from build123d import *

# Parameters (mm, degrees)
SKETCH1_W           = 32.9
SKETCH1_H           = 22.4
BOSS_EXTRUDE1_DEPTH = 5
SKETCH2_R           = 1.2
SKETCH2_W           = 22.9
SKETCH2_H           = 12.4
CUT_EXTRUDE2_DEPTH  = 5
SKETCH3_W           = 22.996888994
SKETCH3_H           = 5
BOSS_EXTRUDE2_DEPTH = 12.3
SKETCH4_R           = 1.2
CUT_EXTRUDE3_DEPTH  = 5
SKETCH6_W           = 5
SKETCH6_H           = 5
SKETCH6_W_2         = 4.903111006
BOSS_EXTRUDE3_DEPTH = 12.3
SKETCH8_W           = 17.3
SKETCH8_H           = 4.998204887
BOSS_EXTRUDE4_DEPTH = 3.1
SKETCH9_W           = 17.3
SKETCH9_H           = 5
BOSS_EXTRUDE5_DEPTH = 3.1
SKETCH18_W          = 5
SKETCH18_H          = 12.4
BOSS_EXTRUDE7_DEPTH = 30
SKETCH19_R          = 4.5
CUT_EXTRUDE6_DEPTH  = 30
SKETCH20_R          = 4.5
CUT_EXTRUDE7_DEPTH  = 30
SKETCH10_W          = 5
SKETCH10_H          = 12.4
BOSS_EXTRUDE6_DEPTH = 30
SKETCH21_R          = 4.5
CUT_EXTRUDE8_DEPTH  = 10
SKETCH22_R          = 4.5
CUT_EXTRUDE9_DEPTH  = 10


with BuildPart() as part:
    # Sketch1 → Boss-Extrude1 (new body)
    with BuildSketch(Plane.XY):
        Rectangle(SKETCH1_W, SKETCH1_H)
    extrude(amount=BOSS_EXTRUDE1_DEPTH)

    # Sketch2 → Cut-Extrude2 (cut)
    with BuildSketch(Plane.XY.offset(5)):
        with Locations((13.8, 0)):
            Circle(SKETCH2_R)
        with Locations((-13.8, 0)):
            Circle(SKETCH2_R)
        Rectangle(SKETCH2_W, SKETCH2_H)
    extrude(amount=-CUT_EXTRUDE2_DEPTH, mode=Mode.SUBTRACT)

    # Sketch3 → Boss-Extrude2 (add)
    with BuildSketch(Plane.XY.offset(5)):
        with Locations((0.048444497, 8.7)):
            Rectangle(SKETCH3_W, SKETCH3_H)
        with Locations((0.048444497, -8.7)):
            Rectangle(SKETCH3_W, SKETCH3_H)
    extrude(amount=BOSS_EXTRUDE2_DEPTH)

    # Sketch4 → Cut-Extrude3 (cut)
    with BuildSketch(Plane.XY.offset(17.3)):
        with Locations((0.048444497, 8.7)):
            Circle(SKETCH4_R)
        with Locations((0.048444497, -8.7)):
            Circle(SKETCH4_R)
    extrude(amount=-CUT_EXTRUDE3_DEPTH, mode=Mode.SUBTRACT)

    # Sketch6 → Boss-Extrude3 (add)
    with BuildSketch(Plane.XY.offset(5)):
        with Locations((-13.95, -8.7)):
            Rectangle(SKETCH6_W, SKETCH6_H)
        with Locations((13.998444497, -8.7)):
            Rectangle(SKETCH6_W_2, SKETCH6_H)
    extrude(amount=BOSS_EXTRUDE3_DEPTH)

    # Sketch8 → Boss-Extrude4 (add)
    with BuildSketch(Plane(origin=(16.45, 0, 0), x_dir=(0, 0, -1), z_dir=(1, 0, 0))):
        with Locations((-8.65, -8.700897557)):
            Rectangle(SKETCH8_W, SKETCH8_H)
    extrude(amount=BOSS_EXTRUDE4_DEPTH)

    # Sketch9 → Boss-Extrude5 (add)
    with BuildSketch(Plane.ZY.offset(16.45)):
        with Locations((8.65, -8.7)):
            Rectangle(SKETCH9_W, SKETCH9_H)
    extrude(amount=BOSS_EXTRUDE5_DEPTH)

    # Sketch18 → Boss-Extrude7 (add)
    with BuildSketch(Plane.XZ.offset(11.2)):
        with Locations((-17.05, 8.65)):
            Rectangle(SKETCH18_W, SKETCH18_H)
        with Locations((17.05, 8.65)):
            Rectangle(SKETCH18_W, SKETCH18_H)
    extrude(amount=BOSS_EXTRUDE7_DEPTH)

    # Sketch19 → Cut-Extrude6 (cut)
    with BuildSketch(Plane.ZY.offset(19.55)):
        with Locations((8.65, -34.8)):
            Circle(SKETCH19_R)
    extrude(amount=-CUT_EXTRUDE6_DEPTH, mode=Mode.SUBTRACT)

    # Sketch20 → Cut-Extrude7 (cut)
    with BuildSketch(Plane(origin=(19.55, 0, 0), x_dir=(0, 0, -1), z_dir=(1, 0, 0))):
        with Locations((-8.65, -34.8)):
            Circle(SKETCH20_R)
    extrude(amount=-CUT_EXTRUDE7_DEPTH, mode=Mode.SUBTRACT)

    # Sketch10 → Boss-Extrude6 (add)
    with BuildSketch(Plane.XZ.offset(11.2)):
        with Locations((17.05, 8.65)):
            Rectangle(SKETCH10_W, SKETCH10_H)
        with Locations((-17.05, 8.65)):
            Rectangle(SKETCH10_W, SKETCH10_H)
    extrude(amount=BOSS_EXTRUDE6_DEPTH)

    # Sketch21 → Cut-Extrude8 (cut)
    with BuildSketch(Plane(origin=(19.55, 0, 0), x_dir=(0, 0, -1), z_dir=(1, 0, 0))):
        with Locations((-8.65, -34.8)):
            Circle(SKETCH21_R)
    extrude(amount=-CUT_EXTRUDE8_DEPTH, mode=Mode.SUBTRACT)

    # Sketch22 → Cut-Extrude9 (cut)
    with BuildSketch(Plane(origin=(-14.55, 0, 0), x_dir=(0, 0, -1), z_dir=(1, 0, 0))):
        with Locations((-8.65, -34.8)):
            Circle(SKETCH22_R)
    extrude(amount=-CUT_EXTRUDE9_DEPTH, mode=Mode.SUBTRACT)


solid = part.part
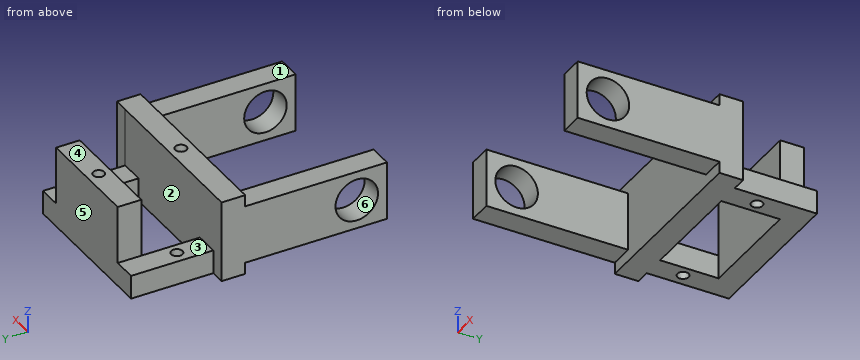
Read the model definition and answer for the solid it produces. Units are mm, in the model's axes. Face numbers are marked on the shaded views. A direction names the side the tool comes from. Round coordinates to 2 decimals unless told otherwise and drop trailing zeros. Write each loop counter-clockwise with the first axis right and the second up, starting at its lowest first coordinate (ties: lowest second). Pieces come first, ordered by that corner, then holes. Notation, with made-up numbers: (-25.5, 63.25) - (-3.5, 63.25) arc R23 cw to (-3.5, 84.25) - close; hole circle Ø7 at (27, 15). An arc over 180 degrees is marked (long way). Use a Markdown table: item, result.
(1) The part is cut by section A-A (y = 5.5). Write down the section's boundary in (x, z).
Reported:
| item | result |
|---|---|
| outline | (-16.45, 0) - (-11.45, 0) - (-11.45, 5) - (-16.45, 5) - close; (11.45, 0) - (16.45, 0) - (16.45, 5) - (11.45, 5) - close |
(2) The part is cut by section D-D (z = 1.75). Write down the section's boundary in (x, y), then the cut area to 3 significant figures.
Reported:
| item | result |
|---|---|
| outline | (-19.55, -11.2) - (19.55, -11.2) - (19.55, -6.2) - (16.45, -6.2) - (16.45, 11.2) - (-16.45, 11.2) - (-16.45, -6.2) - (-19.55, -6.2) - close; hole circle Ø2.4 at (-13.8, 0); hole (-11.45, -6.2) - (11.45, -6.2) - (11.45, 6.2) - (-11.45, 6.2) - close; hole circle Ø2.4 at (13.8, 0) |
| area | 475 mm2 |
(3) The part is cut by section C-C (x = -8). Write down the section's boundary in (y, z).
Reported:
| item | result |
|---|---|
| outline | (-11.2, 0) - (-6.2, 0) - (-6.2, 17.3) - (-11.2, 17.3) - close; (6.2, 0) - (11.2, 0) - (11.2, 17.3) - (6.2, 17.3) - close |
(4) The mould has two halves that part along Y. Classify the marked faces 4, 5 and 6: released by +Y, released by -Y, zero draft, split by the parting line, or undercut.
Reported:
| item | result |
|---|---|
| face 4 | zero draft |
| face 5 | released by +Y |
| face 6 | undercut |
(5) Each of these flat-tipped pins is pushed along its axis until it touches: pin 1 Ø5.5 at (x, y) = (17, -20) entering from -Z; pin 2 Ø2.5 at (y, z) = (9, 10) entering from +X; pin 3 Ø3 at (x, z) = (-2, 12) entering from -Y. Where does it stop, or does it pass through?
Reported:
| item | result |
|---|---|
| pin 1 | z = 2.45 |
| pin 2 | x = 11.55 |
| pin 3 | y = -11.2 |
(6) Which of the six approach directions +Z, -Z, +X, -X, +Y, -Y give full straight-line access (tool end or side, diameter ignored) to the marked faces 1, 2 and 3?
Reported:
| item | result |
|---|---|
| face 1 | +Z, +X, -X, -Y |
| face 2 | +Z |
| face 3 | +Z, -X, +Y |
(7) Straight lines are drawn through the part: line 1 along Y through (x, z) = (-4.5, 12.25); line 2 along Y through (x, z) = (-16.2, 8.65); line 3 along X through (y, z) = (-19.5, 5.25). For each, find the intervals that lie inside material, in ascending order. Write a range as [from, to].
Reported:
| item | result |
|---|---|
| line 1 | [-11.2, -6.2], [6.2, 11.2] |
| line 2 | [-41.2, -39.3], [-30.3, -6.2] |
| line 3 | [-19.55, -14.55], [14.55, 19.55] |
(8) The part is cut by section B-B (y = 0). Write down the section's boundary in (x, z).
Reported:
| item | result |
|---|---|
| outline | (-16.45, 0) - (-15, 0) - (-15, 5) - (-16.45, 5) - close; (-12.6, 0) - (-11.45, 0) - (-11.45, 5) - (-12.6, 5) - close; (11.45, 0) - (12.6, 0) - (12.6, 5) - (11.45, 5) - close; (15, 0) - (16.45, 0) - (16.45, 5) - (15, 5) - close |
